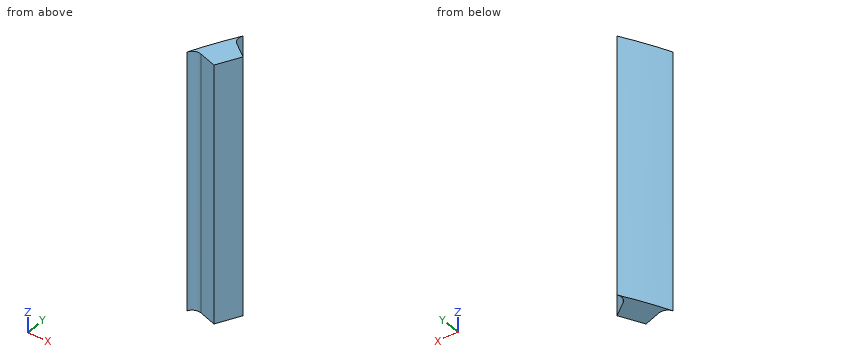
from build123d import *

# Parameters (mm, degrees)
BOSS_EXTRUDE1_DEPTH = 30


with BuildPart() as part:
    # Sketch2 → Boss-Extrude1 (new body)
    with BuildSketch(Plane(origin=(0, 0, -30), x_dir=(-1, 0, 0), z_dir=(0, 0, -1))):
        with BuildLine():
            Line((44.571295977, 20.637196951), (42.558292386, 20.001043701))
            Line((42.558292386, 20.001043701), (41.196320887, 22.674063274))
            Line((41.196320887, 22.674063274), (42.8941935, 23.92869589))
            ThreePointArc((42.8941935, 23.92869589), (43.279434932, 24.531672134), (43.163162714, 25.237697687))
            ThreePointArc((43.163162714, 25.237697687), (44.550326209, 22.699524987), (45.788396813, 20.085385664))
            ThreePointArc((45.788396813, 20.085385664), (45.285553237, 20.594443273), (44.571295977, 20.637196951))
        make_face()
    extrude(amount=-BOSS_EXTRUDE1_DEPTH)


solid = part.part
Read the model definition and answer for the solid it produces. Units are mm, in the model's axes. Coordinates: 2 decimals unless noted, no trailing zeros. Write each loop counter-clockwise with the first axis right and the second up, starting at its lowest first coordinate (ties: lowest second). Pieces come first, ordered by that corner, then holes. Notation, with made-up numbers: (43.5, 41) - (56.5, 41) arc R12 cw to (56.5, 63) - close; hole circle Ø9 at (61, 33.5). An arc over 180 degrees is marked (long way). One line per question, with ' | ' between items.
Q1. Find section A-A, the plane z = -2. Write down the section's boundary in (x, y).
Result set:
outline: (-45.79, 20.09) arc R1 cw to (-44.57, 20.64) - (-42.56, 20) - (-41.2, 22.67) - (-42.89, 23.93) arc R1 cw to (-43.16, 25.24) arc R50 ccw to start
Q2. Find section C-C, the plane y = 21.95. Write down the section's boundary in (x, z).
Result set:
outline: (-44.92, -30) - (-41.57, -30) - (-41.57, 0) - (-44.92, 0) - close
Q3. Each of these flat-tipped pins is pushed along its axis until it touches: P1, Ø1, axis at x = -45.5, y = 24, coming from the -Z side; P2, Ø1.5, axis at x = -44, z = -16.5, coming from the +Y side; P3, Ø1, axis at x = -42, z = -13.5, coming from the +Y side; P4, Ø1.5, axis at y = 22, z = -5.5, coming from the -X side. Where does it stop, or does it pass through?
Result set:
P1: through | P2: y = 25.09 | P3: y = 23.64 | P4: x = -45.26
Q4. Consider L1, parallel to Y at x = -42.2, z = -2.25; L2, parallel to Y at x = -45.1, z = -20.5; L3, parallel to X at y = 21.4, z = -13.75. Determine where each line is inside the solid, lowest interval first. Write a range as [from, to].
Result set:
L1: [20.7, 23.42] | L2: [20.66, 21.59] | L3: [-45.19, -41.85]
Q5. Find section B-B, the plane x = -43.65. Write down the section's boundary in (y, z), plus the area to 3 significant figures.
Result set:
outline: (20.35, -30) - (24.39, -30) - (24.39, 0) - (20.35, 0) - close | area: 121 mm^2
